Source: CAD feature listing. Evaluate the final solid. Frame: model axes, mm. Give positions to 0.01 mm unless a question says otherwise; leave off trailing zeros. Order: outer loops, then holes, each group sorted by start corner. A loop starts at its lowest first (then second) coordinate and runs counter-clockwise, first axis right, second up. Notation, with made-up numbers: (5, 9) - (57, 9) arc R32 ccw to (57, 48) - close; hole circle Ø3 at (71, 5). An arc over 180 degrees is marked (long way). One line per item, written item: value. Start each with the question number.
from build123d import *

# Parameters (mm, degrees)
FILLET1_R          = 1
SKETCH3_W          = 22
SKETCH3_H          = 22
CUT_EXTRUDE1_DEPTH = 2934.613813656


with BuildPart() as part:
    # Sweep1: sweep along a path in Sketch1
    with BuildLine(Plane.XY) as sweep1_path:
        Line((0, 0), (0, 1670))
        ThreePointArc((0, 1670), (83.474567362, 1871.525432638), (285, 1955))
        Line((285, 1955), (1845, 1955))
        ThreePointArc((1845, 1955), (2046.525432638, 1871.525432638), (2130, 1670))
        Line((2130, 1670), (2130, 0))
    # Sketch2 → Sweep1 (sweep)
    with BuildSketch(Plane(origin=(0, 0, 0), x_dir=(1, 0, 0), z_dir=(0, 1, 0))):
        Polygon((0, 0), (0, -2), (-4, -2), (-30, -17.011106999), (-30, -15.011106999), (-7.464101615, -2), (-30, -2), (-30, 0), align=None)
    sweep(path=sweep1_path.line)

    # Fillet1
    # the kernel refuses this fillet: 1 mm, written as the material it adds along each edge
    with BuildSketch(Plane(origin=(2134, 1670, 2), x_dir=(-1.0, -6.753186657693947e-15, -1.7725502571054264e-12), z_dir=(0, -1, 0))) as fillet1_piece_1:
        with BuildLine():
            CenterArc((FILLET1_R * 0.267949192429, -FILLET1_R), FILLET1_R, 90, 30)
            Line((-FILLET1_R * 0.232050807569, -FILLET1_R * 0.133974596215), (0, 0))
            Line((0, 0), (FILLET1_R * 0.267949192431, 0))
        make_face()
    extrude(amount=1670)
    with BuildSketch(Plane(origin=(1845, 1670, 2), x_dir=(0, 1, 0), z_dir=(-1, 0, 0))) as fillet1_piece_2:
        with BuildLine():
            CenterArc((289 - FILLET1_R * 0.267949192431, -FILLET1_R), FILLET1_R, 60, 30)
            Line((289 + FILLET1_R * 0.232050807569, -FILLET1_R * 0.133974596215), (289, 0))
            Line((289, 0), (289 - FILLET1_R * 0.267949192431, 0))
        make_face()
    revolve(axis=Axis((1845, 1670, 2), (0, 0, -1)), revolution_arc=90)
    with BuildSketch(Plane(origin=(285, 1959, 2), x_dir=(0, -1, 0), z_dir=(1, 0, 0))) as fillet1_piece_3:
        with BuildLine():
            CenterArc((FILLET1_R * 0.267949192431, -FILLET1_R), FILLET1_R, 90, 30)
            Line((-FILLET1_R * 0.232050807569, -FILLET1_R * 0.133974596215), (0, 0))
            Line((0, 0), (FILLET1_R * 0.267949192431, 0))
        make_face()
    extrude(amount=1560)
    with BuildSketch(Plane(origin=(285, 1670, 2), x_dir=(-1, 0, 0), z_dir=(0, -1, 0))) as fillet1_piece_4:
        with BuildLine():
            CenterArc((289 - FILLET1_R * 0.267949192431, -FILLET1_R), FILLET1_R, 60, 30)
            Line((289 + FILLET1_R * 0.232050807569, -FILLET1_R * 0.133974596216), (289, 0))
            Line((289, 0), (289 - FILLET1_R * 0.267949192431, 0))
        make_face()
    revolve(axis=Axis((285, 1670, 2), (0, 0, -1)), revolution_arc=90)
    with BuildSketch(Plane(origin=(2137.464101615, 1670, 2), x_dir=(1, 0, 0), z_dir=(0, -1, 0)), Plane(origin=(-7.464101615, 0, 2), x_dir=(-1, 0, 0), z_dir=(0, 1, 0))) as fillet1_piece_5:
        with BuildLine():
            CenterArc((FILLET1_R * 3.73205080757, FILLET1_R), FILLET1_R, 120, 150)
            Line((FILLET1_R * 3.23205080757, FILLET1_R * 1.86602540378), (0, 0))
            Line((0, 0), (FILLET1_R * 3.73205080757, 0))
        make_face()
    extrude(amount=1670)
    with BuildSketch(Plane(origin=(1845, 1670, 2), x_dir=(0, 1, 0), z_dir=(-1, 0, 0))) as fillet1_piece_6:
        with BuildLine():
            CenterArc((292.464101615 + FILLET1_R * 3.73205080757, -FILLET1_R), FILLET1_R, 90, 150)
            Line((292.464101615 + FILLET1_R * 3.23205080757, -FILLET1_R * 1.86602540378), (292.464101615, 0))
            Line((292.464101615, 0), (292.464101615 + FILLET1_R * 3.73205080757, 0))
        make_face()
    revolve(axis=Axis((1845, 1670, 2), (0, 0, -1)), revolution_arc=90)
    with BuildSketch(Plane(origin=(285, 1962.464101615, 2), x_dir=(0, 1, 0), z_dir=(1, 0, 0))) as fillet1_piece_7:
        with BuildLine():
            CenterArc((FILLET1_R * 3.73205080757, FILLET1_R), FILLET1_R, 120, 150)
            Line((FILLET1_R * 3.23205080757, FILLET1_R * 1.86602540378), (0, 0))
            Line((0, 0), (FILLET1_R * 3.73205080757, 0))
        make_face()
    extrude(amount=1560)
    with BuildSketch(Plane(origin=(285, 1670, 2), x_dir=(-1, 0, 0), z_dir=(0, -1, 0))) as fillet1_piece_8:
        with BuildLine():
            CenterArc((292.464101615 + FILLET1_R * 3.73205080757, -FILLET1_R), FILLET1_R, 90, 150)
            Line((292.464101615 + FILLET1_R * 3.23205080757, -FILLET1_R * 1.86602540378), (292.464101615, 0))
            Line((292.464101615, 0), (292.464101615 + FILLET1_R * 3.73205080757, 0))
        make_face()
    revolve(axis=Axis((285, 1670, 2), (0, 0, -1)), revolution_arc=90)
    with BuildSketch(Plane(origin=(-4, 0, 2), x_dir=(-0.8660254037844416, 0, 0.499999999999995), z_dir=(0, 1, 0))) as fillet1_piece_9:
        with BuildLine():
            CenterArc((FILLET1_R * 0.267949192431, FILLET1_R), FILLET1_R, 240, 30)
            Line((-FILLET1_R * 0.232050807569, FILLET1_R * 0.133974596216), (0, 0))
            Line((0, 0), (FILLET1_R * 0.267949192431, 0))
        make_face()
    extrude(amount=1670)
    # the kernel refuses this fillet: 1 mm, written as the material it takes off along each edge
    with BuildSketch(Plane(origin=(2160, 1670, 15.011106999), x_dir=(-0.8660254037844758, -7.797908269406777e-15, -0.49999999999993566), z_dir=(0, -1, 0)), Plane(origin=(-30, -1.443375673, 15.011106999), x_dir=(0.8660254037844414, 0, -0.4999999999999953), z_dir=(0, 1, 0))) as fillet1_2_piece_1:
        with BuildLine():
            CenterArc((FILLET1_R * 0.57735026919, -FILLET1_R), FILLET1_R, 90, 60)
            Line((-FILLET1_R * 0.288675134595, -FILLET1_R * 0.5), (0, 0))
            Line((0, 0), (FILLET1_R * 0.57735026919, 0))
        make_face()
    extrude(amount=1671.443375673, mode=Mode.SUBTRACT)
    with BuildSketch(Plane(origin=(1845, 1670, 15.011106999), x_dir=(0, 1, 0), z_dir=(-1, 0, 0))) as fillet1_2_piece_2:
        with BuildLine():
            CenterArc((315 - FILLET1_R, -FILLET1_R * 0.57735026919), FILLET1_R, 0, 60)
            Line((315 - FILLET1_R * 0.5, FILLET1_R * 0.288675134595), (315, 0))
            Line((315, 0), (315, -FILLET1_R * 0.57735026919))
        make_face()
    revolve(axis=Axis((1845, 1670, 15.011106999), (0, 0, -1)), revolution_arc=90, mode=Mode.SUBTRACT)
    with BuildSketch(Plane(origin=(285, 1985, 15.011106999), x_dir=(0, 0, 1), z_dir=(1, 0, 0))) as fillet1_2_piece_3:
        with BuildLine():
            CenterArc((FILLET1_R * 0.57735026919, FILLET1_R), FILLET1_R, 210, 60)
            Line((-FILLET1_R * 0.288675134595, FILLET1_R * 0.5), (0, 0))
            Line((0, 0), (FILLET1_R * 0.57735026919, 0))
        make_face()
    extrude(amount=1560, mode=Mode.SUBTRACT)
    with BuildSketch(Plane(origin=(285, 1670, 15.011106999), x_dir=(-1, 0, 0), z_dir=(0, -1, 0))) as fillet1_2_piece_4:
        with BuildLine():
            CenterArc((315 - FILLET1_R, -FILLET1_R * 0.57735026919), FILLET1_R, 0, 60)
            Line((315, -FILLET1_R * 0.57735026919), (315, 0))
            Line((315, 0), (315 - FILLET1_R * 0.5, FILLET1_R * 0.288675134595))
        make_face()
    revolve(axis=Axis((285, 1670, 15.011106999), (0, 0, -1)), revolution_arc=90, mode=Mode.SUBTRACT)
    with BuildSketch(Plane(origin=(2160, 1670, 17.011106999), x_dir=(-0.8660254037844523, 0, -0.4999999999999764), z_dir=(0, -1, 0))) as fillet1_2_piece_5:
        with BuildLine():
            CenterArc((FILLET1_R * 1.73205080757, FILLET1_R), FILLET1_R, 150, 120)
            Line((FILLET1_R * 0.866025403784, FILLET1_R * 1.5), (0, 0))
            Line((0, 0), (FILLET1_R * 1.73205080757, 0))
        make_face()
    extrude(amount=1674.330127019, mode=Mode.SUBTRACT)
    with BuildSketch(Plane(origin=(1845, 1670, 17.011106999), x_dir=(0, 1, 0), z_dir=(-1, 0, 0))) as fillet1_2_piece_6:
        with BuildLine():
            CenterArc((315 - FILLET1_R, FILLET1_R * 1.73205080757), FILLET1_R, 240, 120)
            Line((315, FILLET1_R * 1.73205080757), (315, 0))
            Line((315, 0), (315 - FILLET1_R * 1.5, FILLET1_R * 0.866025403784))
        make_face()
    revolve(axis=Axis((1845, 1670, 17.011106999), (0, 0, -1)), revolution_arc=90, mode=Mode.SUBTRACT)
    with BuildSketch(Plane(origin=(285, 1985, 17.011106999), x_dir=(0, -0.8660254037844523, -0.4999999999999764), z_dir=(1, 0, 0))) as fillet1_2_piece_7:
        with BuildLine():
            CenterArc((FILLET1_R * 1.73205080757, FILLET1_R), FILLET1_R, 150, 120)
            Line((FILLET1_R * 0.866025403784, FILLET1_R * 1.5), (0, 0))
            Line((0, 0), (FILLET1_R * 1.73205080757, 0))
        make_face()
    extrude(amount=1560, mode=Mode.SUBTRACT)
    with BuildSketch(Plane(origin=(285, 1670, 17.011106999), x_dir=(-1, 0, 0), z_dir=(0, -1, 0))) as fillet1_2_piece_8:
        with BuildLine():
            CenterArc((315 - FILLET1_R, FILLET1_R * 1.73205080757), FILLET1_R, 240, 120)
            Line((315, FILLET1_R * 1.73205080757), (315, 0))
            Line((315, 0), (315 - FILLET1_R * 1.5, FILLET1_R * 0.866025403784))
        make_face()
    revolve(axis=Axis((285, 1670, 17.011106999), (0, 0, -1)), revolution_arc=90, mode=Mode.SUBTRACT)
    with BuildSketch(Plane(origin=(-30, -4.330127019, 17.011106999), x_dir=(0, 0, -1), z_dir=(0, 1, 0))) as fillet1_2_piece_9:
        with BuildLine():
            CenterArc((FILLET1_R * 1.73205080757, -FILLET1_R), FILLET1_R, 90, 120)
            Line((FILLET1_R * 0.866025403784, -FILLET1_R * 1.5), (0, 0))
            Line((0, 0), (FILLET1_R * 1.73205080757, 0))
        make_face()
    extrude(amount=1674.330127019, mode=Mode.SUBTRACT)

    # Sketch3 → Cut-Extrude1 (cut, through all)
    with BuildSketch(Plane(origin=(0, 0, 0), x_dir=(-1, 0, 0), z_dir=(0, 0, -1))):
        with Locations((-1415, 1970)):
            Rectangle(SKETCH3_W, SKETCH3_H)
        with Locations((-715, 1970)):
            Rectangle(SKETCH3_W, SKETCH3_H)
    extrude(amount=-CUT_EXTRUDE1_DEPTH, mode=Mode.SUBTRACT)


solid = part.part
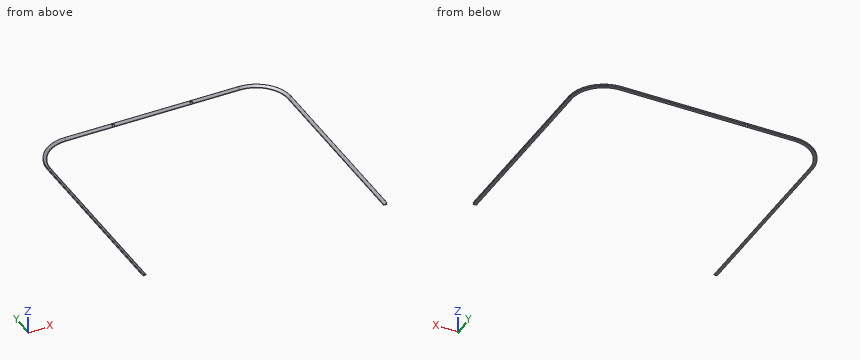
1. Section B-B on z = 6.75. Return the cut outline in (x, y).
2. Section A-A on y = 268.5. Return the cut outline in (x, z), then the cut area to 3 significant figures.
3. Ray query, L1, parallel to X at y = 485, z = 1.5; L2, parallel to Y at x = 1602, z = 1.5; L3, parallel to X at y = 789, z = 13.5. Return the intervals inside material, ascending.
4. Contact query for flat-ended pins moving along their axis: pin 1 Ø1.6 at (x, z) = (714, 14) entering from -Y; pin 2 Ø5 at (y, z) = (308.5, 4) entering from +X; pin 3 Ø2 at (x, z) = (710, 0.5) entering from -Y; pin 4 Ø1.5 at (y, z) = (734.5, 9) entering from -X. Output: stop coordinate, or through.
5. Section C-C on x = 1341.5. Return the cut outline in (y, z).
Data:
1. outline: (-15.69, 0) - (-12.23, 0) - (-12.23, 1670) arc R297.23 cw to (285, 1967.23) - (704, 1967.23) - (704, 1970.69) - (285, 1970.69) arc R300.69 ccw to (-15.69, 1670) - close; (726, 1967.23) - (1404, 1967.23) - (1404, 1970.69) - (726, 1970.69) - close; (1426, 1967.23) - (1845, 1967.23) arc R297.23 cw to (2142.23, 1670) - (2142.23, 0) - (2145.69, 0) - (2145.69, 1670) arc R300.69 ccw to (1845, 1970.69) - (1426, 1970.69) - close
2. outline: (-30, 0) - (0, 0) - (0, 2) - (-3.73, 2) arc R1 cw to (-4.23, 2.13) - (-28.5, 16.15) arc R1 ccw to (-29.99, 15.43) arc R1 ccw to (-29.5, 14.72) - (-10.7, 3.87) arc R1 cw to (-11.2, 2) - (-30, 2) - close; (2130, 0) - (2160, 0) - (2160, 2) - (2141.2, 2) arc R1 cw to (2140.7, 3.87) - (2159.5, 14.72) arc R1 ccw to (2159.99, 15.43) arc R1 ccw to (2158.5, 16.15) - (2134.23, 2.13) arc R1 cw to (2133.73, 2) - (2130, 2) - close
2. area: 220 mm2
3. L1: x = -30 to 0, 2130 to 2160
3. L2: y = 1955 to 1985
3. L3: x = -27.38 to -23.92, 2153.92 to 2157.38
4. pin 1: stops at y = 1981
4. pin 2: stops at x = 2160
4. pin 3: stops at y = 1955
4. pin 4: stops at x = -20.89
5. outline: (1955, 0) - (1985, 0) - (1985, 2) - (1966.2, 2) arc R1 cw to (1965.7, 3.87) - (1984.5, 14.72) arc R1 ccw to (1984.99, 15.43) arc R1 ccw to (1983.5, 16.15) - (1959.23, 2.13) arc R1 cw to (1958.73, 2) - (1955, 2) - close
